Part model, mm, in its own coordinate system. Round coordinates to 2 decimals unless told otherwise and drop trailing zeros. Order: outer loops, then holes, each group sorted by start corner. A loop starts at its lowest first (then second) coordinate and runs counter-clockwise, first axis right, second up. Notation, with made-up numbers: (65.25, 20) - (74.25, 20) arc R8 ccw to (74.25, 24) - close; hole circle Ø4 at (0.5, 48). An arc over 180 degrees is marked (long way). Return JSON: item names as keys, results as strings. Group by question number.
Item 1: Probe probe 1 along Y at (x, z) = (63.5, -2.2); probe 2 along Y at (x, z) = (35.5, -0.15); probe 3 along X at (y, z) = (-0.5, 1.5). List the from-to ranges inside material, lowest first.
Item 2: Saw through at B-B on z = 1.6. List the corners of the cut face in (x, y), and give its area (3 significant figures).
Item 3: Saw through at A-A on x = 91. List the corners of the cut face in (y, z), and give its area (3 significant figures).
Item 4: Drop flat-ended pins along their axis: pin 1 (1 mm diameter, centred on x = 122.5, z = -2, fed in from +Y); pin 2 (1 mm diameter, centred on x = -130, z = -2.5, fed in from -Y); pin 3 (1.5 mm diameter, centred on x = 66, y = -6, fed in from +Z). Give the stop position or say it passes through.
Item 5: Saw through at C-C on x = -180. List the corners of the cut face in (y, z), and give its area (3 significant figures).
```python
from build123d import *

# Parameters (mm, degrees)
BOSS_EXTRUDE1_DEPTH = 3


with BuildPart() as part:
    # Sketch1 → Boss-Extrude1 (new, symmetric)
    with BuildSketch(Plane.XY):
        with BuildLine():
            Line((157.201895781, -12.998193365), (-195.641912802, -5.498193365))
            ThreePointArc((-195.641912802, -5.498193365), (-203.460999592, 2.917559906), (-194.807193354, 10.472337133))
            Line((-194.807193354, 10.472337133), (-117.387348628, 4.017289292))
            ThreePointArc((-117.387348628, 4.017289292), (-116.726087197, 4.00604626), (-116.069126514, 4.082176062))
            Line((-116.069126514, 4.082176062), (-46.416348736, 16.868518301))
            ThreePointArc((-46.416348736, 16.868518301), (-44.971904292, 17), (-43.527459847, 16.868518301))
            Line((-43.527459847, 16.868518301), (26.125317931, 4.082176062))
            ThreePointArc((26.125317931, 4.082176062), (27.028095708, 4), (27.930873486, 4.082176062))
            Line((27.930873486, 4.082176062), (97.583651264, 16.868518301))
            ThreePointArc((97.583651264, 16.868518301), (99.243881438, 16.997089253), (100.894762375, 16.779174478))
            Line((100.894762375, 16.779174478), (159.238570958, 2.779174478))
            ThreePointArc((159.238570958, 2.779174478), (165.306070677, -6.024208847), (157.201895781, -12.998193365))
        make_face()
        with BuildLine():
            Line((-195.056459955, 7.482710708), (-117.63661523, 1.027662867))
            ThreePointArc((-117.63661523, 1.027662867), (-116.57859694, 1.009674016), (-115.527459847, 1.131481699))
            Line((-115.527459847, 1.131481699), (-45.874682069, 13.917823938))
            ThreePointArc((-45.874682069, 13.917823938), (-44.971904292, 14), (-44.069126514, 13.917823938))
            Line((-44.069126514, 13.917823938), (25.583651264, 1.131481699))
            ThreePointArc((25.583651264, 1.131481699), (27.028095708, 1), (28.472540153, 1.131481699))
            Line((28.472540153, 1.131481699), (98.125317931, 13.917823938))
            ThreePointArc((98.125317931, 13.917823938), (99.162961789, 13.998180783), (100.194762375, 13.861984049))
            Line((100.194762375, 13.861984049), (158.538570958, -0.138015951))
            ThreePointArc((158.538570958, -0.138015951), (162.330758283, -5.640130529), (157.265648973, -9.998870853))
            Line((157.265648973, -9.998870853), (-195.578159611, -2.498870853))
            ThreePointArc((-195.578159611, -2.498870853), (-200.465088855, 2.760974942), (-195.056459955, 7.482710708))
        make_face(mode=Mode.SUBTRACT)
    extrude(amount=BOSS_EXTRUDE1_DEPTH, both=True)


solid = part.part
```
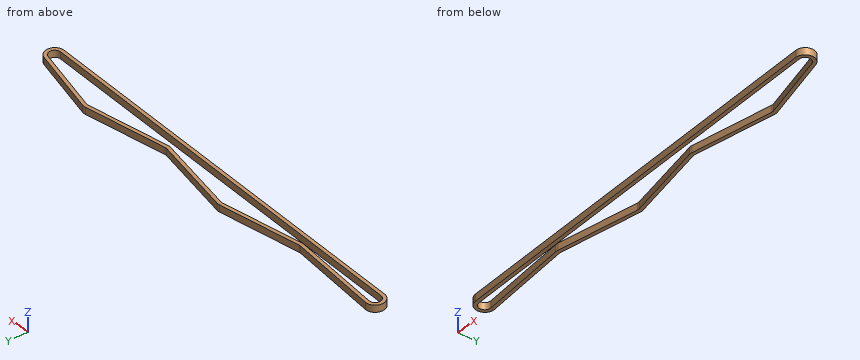
Filled in:
{
 "1": {"probe 1": "y = -11.01 to -8.01, 7.56 to 10.61", "probe 2": "y = -10.41 to -7.41, 2.42 to 5.47", "probe 3": "x = -202.89 to -199.47, 159.55 to 163.99"},
 "2": {"outline": "(-195.64, -5.5) - (157.2, -13) arc R8 ccw to (159.24, 2.78) - (100.89, 16.78) arc R8 ccw to (97.58, 16.87) - (27.93, 4.08) arc R5 cw to (26.13, 4.08) - (-43.53, 16.87) arc R8 ccw to (-46.42, 16.87) - (-116.07, 4.08) arc R5 cw to (-117.39, 4.02) - (-194.81, 10.47) arc R8 ccw (long way) to start; hole (-195.58, -2.5) - (157.27, -10) arc R5 ccw to (158.54, -0.14) - (100.19, 13.86) arc R5 ccw to (98.13, 13.92) - (28.47, 1.13) arc R8 cw to (25.58, 1.13) - (-44.07, 13.92) arc R5 ccw to (-45.87, 13.92) - (-115.53, 1.13) arc R8 cw to (-117.64, 1.03) - (-195.06, 7.48) arc R5 ccw (long way) to start", "area": "2,260 mm^2"},
 "3": {"outline": "(-11.59, -3) - (-8.59, -3) - (-8.59, 3) - (-11.59, 3) - close; (12.61, -3) - (15.66, -3) - (15.66, 3) - (12.61, 3) - close", "area": "36.3 mm^2"},
 "4": {"pin 1": "stops at y = 11.71", "pin 2": "stops at y = -6.9", "pin 3": "passes through"},
 "5": {"outline": "(-5.83, -3) - (-2.83, -3) - (-2.83, 3) - (-5.83, 3) - close; (6.23, -3) - (9.24, -3) - (9.24, 3) - (6.23, 3) - close", "area": "36.1 mm^2"}
}
